Geometry check sheet. Reference: the model listing, model coordinates, mm. A direction names the side the tool comes from. Give positions to 0.01 mm unless a question says otherwise; leave off trailing zeros. Order: outer loops, then holes, each group sorted by start corner. A loop starts at its lowest first (then second) coordinate and runs counter-clockwise, first axis right, second up.
from build123d import *
from OCP.BRepFilletAPI import BRepFilletAPI_MakeChamfer

# Parameters (mm, degrees)
BOSS_EXTRU_1_DEPTH           = 4
BOSS_EXTRU_1_DRAFT           = 3
ESQUISSE1_W                  = 190.5
ESQUISSE1_H                  = 91.5
BOSS_EXTRU_1_PROFILE_2_DEPTH = 4
BOSS_EXTRU_1_PROFILE_2_DRAFT = 3
ESQUISSE1_4_W                = 190.5
ESQUISSE1_4_H                = 91.5
BOSS_EXTRU_2_DEPTH           = 2
CHANFREIN1_SIZE              = 0.528377251
CHANFREIN1_SIZE_2            = 0.5
CHANFREIN2_SIZE              = 0.528377251
CHANFREIN2_SIZE_2            = 0.5


with BuildPart() as part:
    # Esquisse1 → Boss.-Extru.1 (with draft: the straight prism first)
    with BuildSketch(Plane.XY):
        with BuildLine():
            Line((-1, -98.5), (191.5, -98.5))
            ThreePointArc((191.5, -98.5), (195.742640687, -96.742640687), (197.5, -92.5))
            Line((197.5, -92.5), (197.5, 1))
            ThreePointArc((197.5, 1), (195.742640687, 5.242640687), (191.5, 7))
            Line((191.5, 7), (-1, 7))
            ThreePointArc((-1, 7), (-5.242640687, 5.242640687), (-7, 1))
            Line((-7, 1), (-7, -92.5))
            ThreePointArc((-7, -92.5), (-5.242640687, -96.742640687), (-1, -98.5))
        make_face()
        with BuildLine():
            Line((-1, -96.5), (191.5, -96.5))
            ThreePointArc((191.5, -96.5), (194.328427125, -95.328427125), (195.5, -92.5))
            Line((195.5, -92.5), (195.5, 1))
            ThreePointArc((195.5, 1), (194.328427125, 3.828427125), (191.5, 5))
            Line((191.5, 5), (-1, 5))
            ThreePointArc((-1, 5), (-3.828427125, 3.828427125), (-5, 1))
            Line((-5, 1), (-5, -92.5))
            ThreePointArc((-5, -92.5), (-3.828427125, -95.328427125), (-1, -96.5))
        make_face(mode=Mode.SUBTRACT)
    extrude(amount=BOSS_EXTRU_1_DEPTH)
    # Boss.-Extru.1: the draft: its side faces are tilted about the plane it starts from
    boss_extru_1_sides = [part.faces().sort_by_distance(p)[0] for p in [
        (-5.242640687, -96.742640687, 2),
        (95.25, -98.5, 2),
        (195.742640687, -96.742640687, 2),
        (197.5, -45.75, 2),
        (195.742640687, 5.242640687, 2),
        (95.25, 7, 2),
        (-5.242640687, 5.242640687, 2),
        (-7, -45.75, 2),
        (-5, -45.75, 2),
        (-3.828427125, 3.828427125, 2),
        (95.25, 5, 2),
        (194.328427125, 3.828427125, 2),
        (195.5, -45.75, 2),
        (194.328427125, -95.328427125, 2),
        (95.25, -96.5, 2),
        (-3.828427125, -95.328427125, 2),
    ]]
    draft(boss_extru_1_sides, Plane.XY, BOSS_EXTRU_1_DRAFT)



with BuildPart() as body_2:
    # Esquisse1 → Boss.-Extru.1 profile 2 (with draft: the straight prism first)
    with BuildSketch(Plane.XY):
        with BuildLine():
            Line((-1, -93.5), (191.5, -93.5))
            ThreePointArc((191.5, -93.5), (192.207106781, -93.207106781), (192.5, -92.5))
            Line((192.5, -92.5), (192.5, 1))
            ThreePointArc((192.5, 1), (192.207106781, 1.707106781), (191.5, 2))
            Line((191.5, 2), (-1, 2))
            ThreePointArc((-1, 2), (-1.707106781, 1.707106781), (-2, 1))
            Line((-2, 1), (-2, -92.5))
            ThreePointArc((-2, -92.5), (-1.707106781, -93.207106781), (-1, -93.5))
        make_face()
        with Locations((95.25, -45.75)):
            Rectangle(ESQUISSE1_W, ESQUISSE1_H, mode=Mode.SUBTRACT)
    extrude(amount=BOSS_EXTRU_1_PROFILE_2_DEPTH)
    # Boss.-Extru.1 profile 2: the draft: its side faces are tilted about the plane it starts from
    boss_extru_1_profile_2_sides = [body_2.faces().sort_by_distance(p)[0] for p in [
        (-1.707106781, -93.207106781, 2),
        (95.25, -93.5, 2),
        (192.207106781, -93.207106781, 2),
        (192.5, -45.75, 2),
        (192.207106781, 1.707106781, 2),
        (95.25, 2, 2),
        (-1.707106781, 1.707106781, 2),
        (-2, -45.75, 2),
        (95.25, 0, 2),
        (190.5, -45.75, 2),
        (95.25, -91.5, 2),
        (0, -45.75, 2),
    ]]
    draft(boss_extru_1_profile_2_sides, Plane.XY, BOSS_EXTRU_1_PROFILE_2_DRAFT)


with BuildPart() as part_1:
    add(part.part)

    add(body_2.part)  # Boss.-Extru.2 merges body 2
    # Esquisse1<4> → Boss.-Extru.2 (add)
    with BuildSketch(Plane.XY):
        with BuildLine():
            Line((-1, -98.5), (191.5, -98.5))
            ThreePointArc((191.5, -98.5), (195.742640687, -96.742640687), (197.5, -92.5))
            Line((197.5, -92.5), (197.5, 1))
            ThreePointArc((197.5, 1), (195.742640687, 5.242640687), (191.5, 7))
            Line((191.5, 7), (-1, 7))
            ThreePointArc((-1, 7), (-5.242640687, 5.242640687), (-7, 1))
            Line((-7, 1), (-7, -92.5))
            ThreePointArc((-7, -92.5), (-5.242640687, -96.742640687), (-1, -98.5))
        make_face()
        with Locations((95.25, -45.75)):
            Rectangle(ESQUISSE1_4_W, ESQUISSE1_4_H, mode=Mode.SUBTRACT)
    extrude(amount=-BOSS_EXTRU_2_DEPTH)

    # Chanfrein1
    chanfrein1_edges_1 = [part_1.edges().sort_by_distance(p)[0] for p in [
        (-1.558875197, -93.058875197, 4),
    ]]
    chanfrein1_side_1 = [part_1.faces().sort_by_distance(p)[0] for p in [
        (-1.559245268, -93.059245268, 3.990013705),
    ]]
    chanfrein1_edges_2 = [part_1.edges().sort_by_distance(p)[0] for p in [
        (-1.790368883, -45.75, 4),
    ]]
    chanfrein1_side_2 = [part_1.faces().sort_by_distance(p)[0] for p in [
        (-1.790892242, -45.75, 3.990013705),
    ]]
    chanfrein1_edges_3 = [part_1.edges().sort_by_distance(p)[0] for p in [
        (95.25, -93.290368883, 4),
    ]]
    chanfrein1_side_3 = [part_1.faces().sort_by_distance(p)[0] for p in [
        (95.25, -93.290892242, 3.990013705),
    ]]
    chanfrein1_edges_4 = [part_1.edges().sort_by_distance(p)[0] for p in [
        (192.058875197, -93.058875197, 4),
    ]]
    chanfrein1_side_4 = [part_1.faces().sort_by_distance(p)[0] for p in [
        (192.051804129, -93.051804129, 4),
    ]]
    chanfrein1_edges_5 = [part_1.edges().sort_by_distance(p)[0] for p in [
        (192.290368883, -45.75, 4),
    ]]
    chanfrein1_side_5 = [part_1.faces().sort_by_distance(p)[0] for p in [
        (192.280368883, -45.75, 4),
    ]]
    chanfrein1_edges_6 = [part_1.edges().sort_by_distance(p)[0] for p in [
        (192.058875197, 1.558875197, 4),
    ]]
    chanfrein1_side_6 = [part_1.faces().sort_by_distance(p)[0] for p in [
        (192.051804129, 1.551804129, 4),
    ]]
    chanfrein1_edges_7 = [part_1.edges().sort_by_distance(p)[0] for p in [
        (95.25, 1.790368883, 4),
    ]]
    chanfrein1_side_7 = [part_1.faces().sort_by_distance(p)[0] for p in [
        (95.25, 1.780368883, 4),
    ]]
    chanfrein1_edges_8 = [part_1.edges().sort_by_distance(p)[0] for p in [
        (-1.558875197, 1.558875197, 4),
    ]]
    chanfrein1_side_8 = [part_1.faces().sort_by_distance(p)[0] for p in [
        (-1.551804129, 1.551804129, 4),
    ]]
    chanfrein1 = BRepFilletAPI_MakeChamfer(part_1.part.solid().wrapped)
    for e in chanfrein1_edges_1:
        chanfrein1.Add(CHANFREIN1_SIZE, CHANFREIN1_SIZE_2, e.wrapped, chanfrein1_side_1[0].wrapped)
    for e in chanfrein1_edges_2:
        chanfrein1.Add(CHANFREIN1_SIZE, CHANFREIN1_SIZE_2, e.wrapped, chanfrein1_side_2[0].wrapped)
    for e in chanfrein1_edges_3:
        chanfrein1.Add(CHANFREIN1_SIZE, CHANFREIN1_SIZE_2, e.wrapped, chanfrein1_side_3[0].wrapped)
    for e in chanfrein1_edges_4:
        chanfrein1.Add(CHANFREIN1_SIZE_2, CHANFREIN1_SIZE, e.wrapped, chanfrein1_side_4[0].wrapped)
    for e in chanfrein1_edges_5:
        chanfrein1.Add(CHANFREIN1_SIZE_2, CHANFREIN1_SIZE, e.wrapped, chanfrein1_side_5[0].wrapped)
    for e in chanfrein1_edges_6:
        chanfrein1.Add(CHANFREIN1_SIZE_2, CHANFREIN1_SIZE, e.wrapped, chanfrein1_side_6[0].wrapped)
    for e in chanfrein1_edges_7:
        chanfrein1.Add(CHANFREIN1_SIZE, CHANFREIN1_SIZE_2, e.wrapped, chanfrein1_side_7[0].wrapped)
    for e in chanfrein1_edges_8:
        chanfrein1.Add(CHANFREIN1_SIZE_2, CHANFREIN1_SIZE, e.wrapped, chanfrein1_side_8[0].wrapped)
    add(Compound.cast(chanfrein1.Shape()), mode=Mode.REPLACE)

    # Chanfrein2
    chanfrein2_edges_1 = [part_1.edges().sort_by_distance(p)[0] for p in [
        (-3.976658709, 3.976658709, 4),
    ]]
    chanfrein2_side_1 = [part_1.faces().sort_by_distance(p)[0] for p in [
        (-3.976288638, 3.976288638, 3.990013705),
    ]]
    chanfrein2_edges_2 = [part_1.edges().sort_by_distance(p)[0] for p in [
        (95.25, 5.209631117, 4),
    ]]
    chanfrein2_side_2 = [part_1.faces().sort_by_distance(p)[0] for p in [
        (95.25, 5.209107758, 3.990013705),
    ]]
    chanfrein2_edges_3 = [part_1.edges().sort_by_distance(p)[0] for p in [
        (-5.209631117, -45.75, 4),
    ]]
    chanfrein2_side_3 = [part_1.faces().sort_by_distance(p)[0] for p in [
        (-5.209107758, -45.75, 3.990013705),
    ]]
    chanfrein2_edges_4 = [part_1.edges().sort_by_distance(p)[0] for p in [
        (194.476658709, 3.976658709, 4),
    ]]
    chanfrein2_side_4 = [part_1.faces().sort_by_distance(p)[0] for p in [
        (194.476288638, 3.976288638, 3.990013705),
    ]]
    chanfrein2_edges_5 = [part_1.edges().sort_by_distance(p)[0] for p in [
        (-3.976658709, -95.476658709, 4),
    ]]
    chanfrein2_side_5 = [part_1.faces().sort_by_distance(p)[0] for p in [
        (-3.976288638, -95.476288638, 3.990013705),
    ]]
    chanfrein2_edges_6 = [part_1.edges().sort_by_distance(p)[0] for p in [
        (195.709631117, -45.75, 4),
    ]]
    chanfrein2_side_6 = [part_1.faces().sort_by_distance(p)[0] for p in [
        (195.709107758, -45.75, 3.990013705),
    ]]
    chanfrein2_edges_7 = [part_1.edges().sort_by_distance(p)[0] for p in [
        (95.25, -96.709631117, 4),
    ]]
    chanfrein2_side_7 = [part_1.faces().sort_by_distance(p)[0] for p in [
        (95.25, -96.709107758, 3.990013705),
    ]]
    chanfrein2_edges_8 = [part_1.edges().sort_by_distance(p)[0] for p in [
        (194.476658709, -95.476658709, 4),
    ]]
    chanfrein2_side_8 = [part_1.faces().sort_by_distance(p)[0] for p in [
        (194.476288638, -95.476288638, 3.990013705),
    ]]
    chanfrein2 = BRepFilletAPI_MakeChamfer(part_1.part.solid().wrapped)
    for e in chanfrein2_edges_1:
        chanfrein2.Add(CHANFREIN2_SIZE, CHANFREIN2_SIZE_2, e.wrapped, chanfrein2_side_1[0].wrapped)
    for e in chanfrein2_edges_2:
        chanfrein2.Add(CHANFREIN2_SIZE, CHANFREIN2_SIZE_2, e.wrapped, chanfrein2_side_2[0].wrapped)
    for e in chanfrein2_edges_3:
        chanfrein2.Add(CHANFREIN2_SIZE, CHANFREIN2_SIZE_2, e.wrapped, chanfrein2_side_3[0].wrapped)
    for e in chanfrein2_edges_4:
        chanfrein2.Add(CHANFREIN2_SIZE_2, CHANFREIN2_SIZE, e.wrapped, chanfrein2_side_4[0].wrapped)
    for e in chanfrein2_edges_5:
        chanfrein2.Add(CHANFREIN2_SIZE, CHANFREIN2_SIZE_2, e.wrapped, chanfrein2_side_5[0].wrapped)
    for e in chanfrein2_edges_6:
        chanfrein2.Add(CHANFREIN2_SIZE, CHANFREIN2_SIZE_2, e.wrapped, chanfrein2_side_6[0].wrapped)
    for e in chanfrein2_edges_7:
        chanfrein2.Add(CHANFREIN2_SIZE, CHANFREIN2_SIZE_2, e.wrapped, chanfrein2_side_7[0].wrapped)
    for e in chanfrein2_edges_8:
        chanfrein2.Add(CHANFREIN2_SIZE, CHANFREIN2_SIZE_2, e.wrapped, chanfrein2_side_8[0].wrapped)
    add(Compound.cast(chanfrein2.Shape()), mode=Mode.REPLACE)


solid = part_1.part
Item 1: Sectioned sample at A-A (y = -18). Enter the section's corners in (x, z), and give its area (3 significant figures).
Reported:
outline: (-7, -2) - (0, -2) - (0, 0) - (-0.21, 4) - (-1.29, 4) - (-1.82, 3.47) - (-2, 0) - (-5, 0) - (-5.18, 3.47) - (-5.71, 4) - (-6.79, 4) - (-7, 0) - close; (190.5, -2) - (197.5, -2) - (197.5, 0) - (197.29, 4) - (196.21, 4) - (195.68, 3.47) - (195.5, 0) - (192.5, 0) - (192.32, 3.47) - (191.79, 4) - (190.71, 4) - (190.5, 0) - close
area: 56.1 mm2
Item 2: Set-up check for faces 1 (the conical face through (-5.22, -96.62, 1.97)), 2 (the flat face through (-1.91, -45.1, 1.71)): record each of +Z, -Z, +X, -X, +Y, -Y from which the full face is reachable in a straight line by a thin tool's end or side.
Reported:
face 1: +Z, -X, -Y
face 2: +Z
Item 3: Scan lines: L1, parallel to X at y = -13, z = 0.5; L2, parallel to Y at x = 23, z = 0.5; L3, parallel to Y at x = 17, z = 3.25. Record each from-to range of solid material in increasing order.
Reported:
L1: x = -6.97 to -5.03, -1.97 to -0.03, 190.53 to 192.47, 195.53 to 197.47
L2: y = -98.47 to -96.53, -93.47 to -91.53, 0.03 to 1.97, 5.03 to 6.97
L3: y = -98.33 to -96.67, -93.33 to -91.67, 0.17 to 1.83, 5.17 to 6.83
Item 4: Sectioned sample at C-C (z = 2.5). Enter the section's corners in (x, y), and give its area (3 significant figures).
Reported:
outline: (-6.87, -92.5) arc R5.87 ccw to (-1, -98.37) - (191.5, -98.37) arc R5.87 ccw to (197.37, -92.5) - (197.37, 1) arc R5.87 ccw to (191.5, 6.87) - (-1, 6.87) arc R5.87 ccw to (-6.87, 1) - close; (-1.87, -92.5) arc R0.87 ccw to (-1, -93.37) - (191.5, -93.37) arc R0.87 ccw to (192.37, -92.5) - (192.37, 1) arc R0.87 ccw to (191.5, 1.87) - (-1, 1.87) arc R0.87 ccw to (-1.87, 1) - close; hole (-5.13, -92.5) arc R4.13 ccw to (-1, -96.63) - (191.5, -96.63) arc R4.13 ccw to (195.63, -92.5) - (195.63, 1) arc R4.13 ccw to (191.5, 5.13) - (-1, 5.13) arc R4.13 ccw to (-5.13, 1) - close; hole (-0.13, -91.63) - (190.63, -91.63) - (190.63, 0.13) - (-0.13, 0.13) - close
area: 2,040 mm2
Item 5: Gauge pin test, flat ends, axial feed: pin 1 (1.5 mm diameter, centred on x = 166, z = 3, fed in from +Y); pin 2 (1.5 mm diameter, centred on y = -14, z = 3.5, fed in from +X). Record the tip position at first contact, or that the pin passes through.
Reported:
pin 1: stops at y = 6.88
pin 2: stops at x = 197.36
Item 6: Draft check along Y on faces 3 (the cylindrical face through (-5.196, 5.289, -0.986)), 4 (the flat face through (87, -92, -2)), 5 (the flat face through (95, 3, 0)). Enter one of: released by +Y, released by -Y, zero draft, split by the parting line, or undercut.
Reported:
face 3: released by +Y
face 4: zero draft
face 5: undercut
Item 7: Sectioned sample at B-B (x = 171). Enter the section's corners in (y, z), and give its area (3 significant figures).
Reported:
outline: (-98.5, -2) - (-91.5, -2) - (-91.5, 0) - (-91.71, 4) - (-92.79, 4) - (-93.32, 3.47) - (-93.5, 0) - (-96.5, 0) - (-96.68, 3.47) - (-97.21, 4) - (-98.29, 4) - (-98.5, 0) - close; (0, -2) - (7, -2) - (7, 0) - (6.79, 4) - (5.71, 4) - (5.18, 3.47) - (5, 0) - (2, 0) - (1.82, 3.47) - (1.29, 4) - (0.21, 4) - (0, 0) - close
area: 56.1 mm2
